Source: CAD feature listing. Evaluate the final solid. Frame: model axes, mm. Face numbers are marked on the shaded views. A direction names the side the tool comes from. Give positions to 0.01 mm unless a question says otherwise; leave off trailing zeros. Loops run counter-clockwise (first coordinate to the right, second up) from the corner with the lowest first, then second, coordinate; pieces in that order, holes last. Notation, with made-up numbers: (10.5, 7) -> (56.5, 7) arc R28 cw to (56.5, 29) -> close; hole circle Ø9 at (7.5, 66.25). An arc over 180 degrees is marked (long way). Return JSON: item names as keys, results as strings. Group by question number.
Autodesk Inventor part; units mm, degrees
ref_plane "YZ Plane" through (0, 0, 0) normal (1, 0, 0) x (0, 1, 0)
ref_plane "XZ Plane" through (0, 0, 0) normal (0, 1, 0) x (-1, 0, 0)
ref_plane "XY Plane" through (0, 0, 0) normal (0, 0, 1) x (1, 0, 0)
sketch "Sketch1" plane through (0, 0, 0) normal (0, 0, 1) x (1, 0, 0)
  circle A0 centre (0, 0) radius 4
  circle A1 centre (0, 0) radius 100
  dimension "d0" = 8
  dimension "d1" = 200
extrude "Extrusion1" add sketch "Sketch1" along normal blind 29
fillet "Fillet1" radius 12 2 edges at (-100, 0, 29) (-100, 0, 0)
sketch "Sketch2" plane through (0, 0, 29) normal (0, 0, 1) x (1, 0, 0)
  circle A0 centre (0, 0) radius 88
  line L0 (9.0297, 17.8456) -> (73.5273, -14.7895)
  line L1 (19.5363, -4.2815) -> (69.0295, -29.3245)
  arc A1 (19.5363, -4.2815) -> (9.0297, 17.8456) centre (0, 0) ccw
  arc A2 (69.0295, -29.3245) -> (73.5273, -14.7895) centre (0, 0) ccw
  line L2 (13.4761, 14.7782) -> (59.9105, 45.119)
  arc A3 (13.4761, 14.7782) -> (-10.9399, 16.7427) centre (0, 0) ccw
  arc A4 (59.9105, 45.119) -> (49.5718, 56.2818) centre (0, 0) ccw
  line L3 (-10.9399, 16.7427) -> (49.5718, 56.2818)
  line L4 (-6.0602, 19.0597) -> (-9.119, 74.4436)
  arc A5 (-6.0602, 19.0597) -> (-19.9696, -1.1029) centre (0, 0) ccw
  arc A6 (-9.119, 74.4436) -> (-23.9556, 71.0713) centre (0, 0) ccw
  line L5 (-19.9696, -1.1029) -> (-23.9556, 71.0713)
  line L6 (-19.5363, 4.2815) -> (-69.0295, 29.3245)
  arc A7 (-19.5363, 4.2815) -> (-9.0297, -17.8456) centre (0, 0) ccw
  arc A8 (-69.0295, 29.3245) -> (-73.5273, 14.7895) centre (0, 0) ccw
  line L7 (-9.0297, -17.8456) -> (-73.5273, 14.7895)
  line L8 (-13.4761, -14.7782) -> (-59.9105, -45.119)
  arc A9 (-13.4761, -14.7782) -> (10.9399, -16.7427) centre (0, 0) ccw
  arc A10 (-59.9105, -45.119) -> (-49.5718, -56.2818) centre (0, 0) ccw
  line L9 (10.9399, -16.7427) -> (-49.5718, -56.2818)
  line L10 (6.0602, -19.0597) -> (9.119, -74.4436)
  arc A11 (6.0602, -19.0597) -> (19.9696, 1.1029) centre (0, 0) ccw
  arc A12 (9.119, -74.4436) -> (23.9556, -71.0713) centre (0, 0) ccw
  line L11 (19.9696, 1.1029) -> (23.9556, -71.0713)
  circle A13 centre (0, 0) radius 4
  circle A14 centre (0, 0) radius 75
  dimension "d7" = 15
  dimension "d8" = 75
  dimension "d9" = 20
  dimension "d12" = 360
extrude "Extrusion2" cut sketch "Sketch2" against normal through all contours A1 A11 A9 A7 A5 A3 | L2 A14 L0 | L4 A14 L3 | A14 L11 L1 | L6 A14 L5 | A14 L9 L10 | L8 A14 L7
sketch "Sketch3" plane through (0, 0, 29) normal (0, 0, 1) x (1, 0, 0)
  circle A0 centre (0, 0) radius 25
  circle A1 centre (0, 0) radius 20
  dimension "d16" = 50
extrude "Extrusion3" add sketch "Sketch3" against normal blind 29
sketch "Sketch4" plane through (0, 0, 29) normal (0, 0, 1) x (1, 0, 0)
  circle A0 centre (0, 0) radius 20
  circle A1 centre (0, 0) radius 4
  dimension "d19" = 8
extrude "Extrusion4" add sketch "Sketch4" against normal blind 29
sketch "Sketch5" plane through (0, 0, 29) normal (0, 0, 1) x (1, 0, 0)
  circle A0 centre (0, 0) radius 4
  circle A1 centre (0, 0) radius 11
  dimension "d22" = 22
extrude "Extrusion5" cut sketch "Sketch5" against normal blind 10
sketch "Sketch7" plane through (0, 0, 0) normal (0, 0, -1) x (-1, 0, 0)
  circle A0 centre (0, 0) radius 4
  circle A1 centre (0, 0) radius 11
  dimension "d25" = 22
extrude "Extrusion6" cut sketch "Sketch7" against normal blind 10
properties part number "Scooter Wheel" material "Rubber"
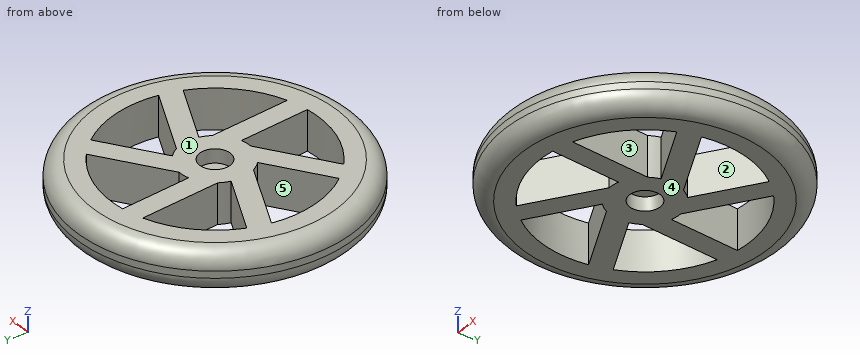
1) Cut plane A-A on z = 24.75. Return loops of the section in (x, y), then the cut area to 3 significant figures.
2) Cut plane B-B on y = 0. Return loops of the section in (x, z), then the cut area to 3 significant figures.
3) Contact query for flat-ended pins moving along their axis: P1, Ø1, axis at y = -70.5, z = 22.5, coming from the +X side; P2, Ø3, axis at x = 60, z = 4, coming from the -Y side; P3, Ø9, axis at x = 0, y = 0, coming from the -Z side; P4, Ø17.5, axis at x = -4.5, y = 3.5, coming from the +Z side. Output: stop coordinate, or through.
4) Cut plane C-C on x = -29.5. Count the separate pieces of the cut face and the enclosed holes in it, then the cut area to 3 significant figures.
5) Mould query, pull axis X, two halves, no side actions, for the marked faces 3, 4 and 5. Classes: released by +X, released by -X, zero draft, split by the parting line, or undercut.
6) Material intervals for line 1 (Y direction, x = 0, z = 13); line 2 (X direction, y = 12.5, z = 21.25); line 3 (X direction, y = -1.5, z = 10.25) (3 decimals), sorted ascending.
7) Reachability of the marked faces 1 and 2 from +Z, -Z, +X, -X, +Y, -Y: full face, straight path, thin tool, end or side. Return the list, or none.
Calculated:
{
 "1": {"outline": "circle Ø194.32 at (0, 0); hole (-73.53, 14.79) arc R75 ccw to (-59.91, -45.12) -> (-17.77, -17.58) arc R25 cw to (-22.41, -11.07) -> close; hole (-69.03, 29.32) -> (-24.11, 6.6) arc R25 cw to (-20.8, 13.87) -> (-23.96, 71.07) arc R75 ccw to start; hole (-49.57, -56.28) arc R75 ccw to (9.12, -74.44) -> (6.34, -24.18) arc R25 cw to (-1.62, -24.95) -> close; hole circle Ø22 at (0, 0); hole (-9.12, 74.44) -> (-6.34, 24.18) arc R25 cw to (1.62, 24.95) -> (49.57, 56.28) arc R75 ccw to start; hole (17.77, 17.58) arc R25 cw to (22.41, 11.07) -> (73.53, -14.79) arc R75 ccw to (59.91, 45.12) -> close; hole (20.8, -13.87) -> (23.96, -71.07) arc R75 ccw to (69.03, -29.32) -> (24.11, -6.6) arc R25 cw to start", "area": "18,300 mm2"},
 "2": {"outline": "(-100, 12) arc R12 ccw to (-88, 0) -> (-75, 0) -> (-75, 29) -> (-88, 29) arc R12 ccw to (-100, 17) -> close; (-44.3, 0) -> (-11, 0) -> (-11, 10) -> (-4, 10) -> (-4, 19) -> (-11, 19) -> (-11, 29) -> (-44.3, 29) -> close; (4, 10) -> (11, 10) -> (11, 0) -> (44.3, 0) -> (44.3, 29) -> (11, 29) -> (11, 19) -> (4, 19) -> close; (75, 0) -> (88, 0) arc R12 ccw to (100, 12) -> (100, 17) arc R12 ccw to (88, 29) -> (75, 29) -> close", "area": "3,380 mm2"},
 "3": {"P1": "x = 69.65", "P2": "y = -78.04", "P3": "z = 10", "P4": "z = 29"},
 "4": {"separate pieces": "4", "enclosed holes": "0", "area": "2,420 mm2"},
 "5": {"face 3": "undercut", "face 4": "zero draft", "face 5": "undercut"},
 "6": {"line 1": "-100 to -75, -25 to -4, 4 to 25, 75 to 100", "line 2": "-98.43 to -73.95, -69 to -35.78, -21.65 to 21.65, 73.95 to 98.43", "line 3": "-99.86 to -74.985, -41.334 to -3.708, 3.708 to 47.263, 74.985 to 99.86"},
 "7": {"face 1": "+Z, +X, -X, +Y, -Y", "face 2": "+Z, -Z"}
}
